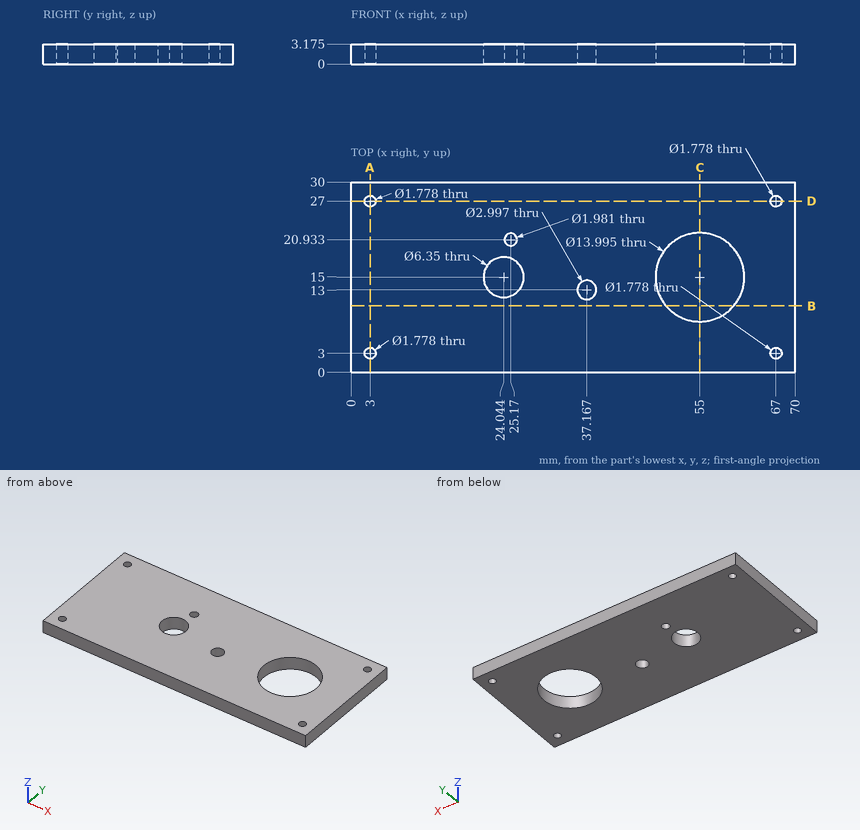
Answer from the drawing. Dimensions are ordinates in mm from the lowest x, y and z of the part. Coordinates: 2 decimals unless noted, no trailing zeros. Order: outer loops, then holes, each group sorted by start corner. A loop starts at its lowest first (then second) coordinate and runs counter-clockwise, first axis right, second up. Notation, with made-up numbers: (35, -20.5) - (51, -20.5) arc R20 ccw to (51, 0.5) - close; hole circle Ø10 at (87.25, -7). An arc over 180 degrees is marked (long way). Put each result on its own line as item: value. Start each with the question number.
1) A flat-ended cylindrical pin translates along its axis: pin 1 (2.5 mm diameter, centred on x = 37.17, y = 13, fed in from -Z). Find the tip coordinate at first contact, or state that the pin passes through.
2) Find section C-C (x = 55). Give the vertices of the cut face in (y, z) (1 decimal).
3) Find section A-A (x = 3). Give the vertices of the cut face in (y, z) (1 decimal).
4) Find section B-B (y = 10.5). Give the vertices of the cut face in (x, z) (1 decimal).
5) Find section D-D (y = 27). Give the vertices of the cut face in (x, z) (1 decimal).
6) Find the intervals of material crossed by line 1 (Y direction, x = 3, z = 1.25); line 2 (X direction, y = 16, z = 2.6) (1 decimal); line 3 (Y direction, x = 55, z = 1.9), in increasing order. Write a range as from..to.
Results list:
1. pin 1: passes through
2. outline: (0, 0) - (8, 0) - (8, 3.2) - (0, 3.2) - close; (22, 0) - (30, 0) - (30, 3.2) - (22, 3.2) - close
3. outline: (0, 0) - (2.1, 0) - (2.1, 3.2) - (0, 3.2) - close; (3.9, 0) - (26.1, 0) - (26.1, 3.2) - (3.9, 3.2) - close; (27.9, 0) - (30, 0) - (30, 3.2) - (27.9, 3.2) - close
4. outline: (0, 0) - (49.6, 0) - (49.6, 3.2) - (0, 3.2) - close; (60.4, 0) - (70, 0) - (70, 3.2) - (60.4, 3.2) - close
5. outline: (0, 0) - (2.1, 0) - (2.1, 3.2) - (0, 3.2) - close; (3.9, 0) - (66.1, 0) - (66.1, 3.2) - (3.9, 3.2) - close; (67.9, 0) - (70, 0) - (70, 3.2) - (67.9, 3.2) - close
6. line 1: y = 0..2.11, 3.89..26.11, 27.89..30
6. line 2: x = 0..21, 27.1..48.1, 61.9..70
6. line 3: y = 0..8, 22..30
